from build123d import *

# Parameters (mm, degrees)
BOSS_EXTRUDE1_DEPTH = 3.175
FILLET1_R           = 5.08
CUT_EXTRUDE2_DEPTH  = 3.175
FILLET2_R           = 5.08
SKETCH4_R           = 3.175
CUT_EXTRUDE3_DEPTH  = 3.175


with BuildPart() as part:
    # Sketch1 → Boss-Extrude1 (new body)
    with BuildSketch(Plane(origin=(0, 0, 0), x_dir=(1, 0, 0), z_dir=(0, 1, 0))):
        Polygon((0, 0), (393.7, 0), (196.85, 340.95420147), align=None)
    extrude(amount=BOSS_EXTRUDE1_DEPTH)

    # Fillet1
    fillet1_edges = [part.edges().sort_by_distance(p)[0] for p in [
        (196.85, 1.5875, -340.95420147),
        (393.7, 1.5875, 0),
        (0, 1.5875, 0),
    ]]
    fillet(fillet1_edges, radius=FILLET1_R)

    # Sketch3 → Cut-Extrude2 (cut)
    with BuildSketch(Plane(origin=(0, 3.175, 0), x_dir=(1, 0, 0), z_dir=(0, 1, 0))):
        with BuildLine():
            Line((389.300590949, 7.62), (210.598153285, 317.14170147))
            ThreePointArc((210.598153285, 317.14170147), (212.184072492, 313.312953811), (212.725, 309.20420147))
            Line((212.725, 309.20420147), (212.725, 0))
            Line((212.725, 0), (384.901181898, 0))
            ThreePointArc((384.901181898, 0), (389.300590949, 2.54), (389.300590949, 7.62))
        make_face()
        with BuildLine():
            Line((210.598153285, 317.14170147), (201.249409051, 333.33420147))
            ThreePointArc((201.249409051, 333.33420147), (196.85, 335.87420147), (192.450590949, 333.33420147))
            Line((192.450590949, 333.33420147), (183.101846715, 317.14170147))
            ThreePointArc((183.101846715, 317.14170147), (196.85, 325.07920147), (210.598153285, 317.14170147))
        make_face()
    extrude(amount=-CUT_EXTRUDE2_DEPTH, mode=Mode.SUBTRACT)

    # Fillet2
    fillet2_edges = [part.edges().sort_by_distance(p)[0] for p in [
        (212.725, 1.5875, 0),
    ]]
    fillet(fillet2_edges, radius=FILLET2_R)

    # Sketch4 → Cut-Extrude3 (cut)
    with BuildSketch(Plane(origin=(0, 3.175, 0), x_dir=(1, 0, 0), z_dir=(0, 1, 0))):
        with Locations((196.028249532, 306.137386971)):
            Circle(SKETCH4_R)
        with Locations((202.256846327, 10.468153673)):
            Circle(SKETCH4_R)
        with Locations((15.397931679, 8.89)):
            Circle(SKETCH4_R)
    extrude(amount=-CUT_EXTRUDE3_DEPTH, mode=Mode.SUBTRACT)


solid = part.part
The listing builds one solid part. Answer for the finished solid, in the listing's coordinates (mm). Coordinates: 2 decimals unless noted, no trailing zeros. Loops run counter-clockwise (first coordinate to the right, second up) from the corner with the lowest first, then second, coordinate; pieces in that order, holes last. Notation, with made-up numbers: (69.25, 10.5) -> (92.25, 10.5) arc R25 cw to (92.25, 33.5) -> close; hole circle Ø9 at (31, 83.5). An arc over 180 degrees is marked (long way). Answer in a Markdown table with one row per item. Add a question column.
1. Consider line 1 (X direction, y = 1.6, z = -8.89) (3 decimals); line 2 (X direction, y = 2.35, z = -307) (3 decimals); line 3 (Z direction, x = 200, y = 2.2). Determine where each line is inside the solid, lowest interval first. Write a range as [from, to].
2. The part is cut by section A-A, the plane x = 96. Write down the section's boundary in (y, z) (3 decimals).
3. The part is cut by section B-B, the plane z = -270. Write down the section's boundary in (x, y) (3 decimals).
Answer below:
| question | item | result |
|---|---|---|
| 1 | line 1 | [5.133, 12.223], [18.573, 199.502], [205.012, 212.725] |
| 1 | line 2 | [177.247, 192.973], [199.084, 212.725] |
| 1 | line 3 | [-324.76, -12.7], [-8.23, 0] |
| 2 | outline | (0, -166.277) -> (3.175, -166.277) -> (3.175, 0) -> (0, 0) -> close |
| 3 | outline | (155.885, 0) -> (212.725, 0) -> (212.725, 3.175) -> (155.885, 3.175) -> close |
